The listing builds one solid part. Answer for the finished solid, in the listing's coordinates (mm). A direction names the side the tool comes from. Coordinates: 2 decimals unless noted, no trailing zeros. Order: outer loops, then holes, each group sorted by start corner. A loop starts at its lowest first (then second) coordinate and runs counter-clockwise, first axis right, second up. Notation, with made-up numbers: (63, 34.5) -> (91, 34.5) arc R11 cw to (91, 42.5) -> close; hole circle Ø11 at (-28, 22.5). An arc over 180 degrees is marked (long way). Write each question's results on one line, items separated by ' | '. Start each with the question number.
(1) The part is cut by section D-D, the plane z = 0.75. Give the vertices of the cut face in (x, y).
(2) The part is cut by section A-A, the plane z = 5.75. Give the vertices of the cut face in (x, y), then the cut area to 3 significant figures.
(3) Determine the mould class of faces 4 (the face through (-0.145, -2.073, 12.387)), 5 (the face through (-0.145, -2.073, -12.313)), 6 (the face through (17.66, -3.13, -0.92)), 7 (the face through (8, -6.35, 7)) for opening direction Y: +Y half, -Y half, draft (parallel to the pull), parting line (faces both ways), or undercut.
(4) Given pin 1 (1.9 mm diameter, centred on x = 18, y = -4, fed in from +Z), flat-ended and moving along its own axis, determine where the tip first touches the part or whether it passes through.
(5) The part is cut by section B-B, the plane x = 0. Give the vertices of the cut face in (y, z).
(6) A tool of negligible diameter and unlimited length cuts with its end or side. For faces 1 (the face through (-14.98, -3.13, 0.42)), 2 (the face through (19, -3, 5.231)), 3 (the face through (19, -3, -4.929)), from which of +Z, -Z, +X, -X, +Y, -Y can it reach the whole face along a straight path? Write none if from no direction.
(7) Straight lines are drawn through the part: L1, parallel to X at y = -1, z = 0.25; L2, parallel to Y at x = 0, z = -13; L3, parallel to Z at x = 9, y = -1. For each, find the intervals that lie inside material, in ascending order.
(8) The part is cut by section C-C, the plane y = -5. Give the vertices of the cut face in (x, z).
```python
from build123d import *

# Parameters (mm, degrees)
F0_R     = 1.7526
F0_R_2   = 9.779
F1_DEPTH = 6.35
F2_R     = 1.11125
F3_DEPTH = 25.4
F4_R     = 2.54
F5_R     = 2.54


with BuildPart() as f1:
    # F0 (on Front) → F1 (new body)
    with BuildSketch(Plane.XZ):
        with BuildLine():
            ThreePointArc((14.1521138842, -4.9292868255), (14.7760579092, -2.4996617102), (14.986, 0))
            ThreePointArc((14.986, 0), (14.7484924114, 2.6574739115), (14.0434979861, 5.2307131745))
            Line((14.0434979861, 5.2307131745), (14.0434979861, -4.9292868255))
            Line((14.0434979861, -4.9292868255), (14.1521138842, -4.9292868255))
        make_face()
        with BuildLine():
            ThreePointArc((14.0434979861, 5.2307131745), (14.7484924114, 2.6574739115), (14.986, 0))
            ThreePointArc((14.986, 0), (14.7760579092, -2.4996617102), (14.1521138842, -4.9292868255))
            Line((14.1521138842, -4.9292868255), (23.0350979861, -4.9292868255))
            Line((23.0350979861, -4.9292868255), (23.0350979861, 5.2307131745))
            Line((23.0350979861, 5.2307131745), (14.0434979861, 5.2307131745))
        make_face()
        with Locations((19.0472979861, 0.1507131745)):
            Circle(F0_R, mode=Mode.SUBTRACT)
        with BuildLine():
            Line((14.0434979861, -4.9292868255), (14.0434979861, 5.2307131745))
            ThreePointArc((14.0434979861, 5.2307131745), (-14.9851437159, -0.1601992956), (14.1521138842, -4.9292868255))
            Line((14.1521138842, -4.9292868255), (14.0434979861, -4.9292868255))
        make_face()
        Circle(F0_R_2, mode=Mode.SUBTRACT)
    extrude(amount=F1_DEPTH)

    # F2 (on Top) → F3 (cut, symmetric)
    with BuildSketch(Plane.XY):
        with Locations((0, -3.175)):
            Circle(F2_R)
    extrude(amount=F3_DEPTH, both=True, mode=Mode.SUBTRACT)

    # F4
    f4_edges = [f1.edges().sort_by_distance(p)[0] for p in [
        (14.043498, -3.175, 5.230713),
    ]]
    fillet(f4_edges, radius=F4_R)

    # F5
    f5_edges = [f1.edges().sort_by_distance(p)[0] for p in [
        (14.152114, -3.175, -4.929287),
    ]]
    fillet(f5_edges, radius=F5_R)


solid = f1.part
```
Established:
1) outline: (-14.97, -6.35) -> (-9.75, -6.35) -> (-9.75, 0) -> (-14.97, 0) -> close; (9.75, -6.35) -> (17.4, -6.35) -> (17.4, 0) -> (9.75, 0) -> close; (20.69, -6.35) -> (23.04, -6.35) -> (23.04, 0) -> (20.69, 0) -> close
2) outline: (-13.84, -6.35) -> (-7.91, -6.35) -> (-7.91, 0) -> (-13.84, 0) -> close; (7.91, -6.35) -> (14.17, -6.35) -> (14.17, 0) -> (7.91, 0) -> close | area: 77.4 mm^2
3) face 4: undercut | face 5: undercut | face 6: draft | face 7: -Y half
4) pin 1: stops at z = 5.23
5) outline: (-6.35, -14.99) -> (-4.29, -14.99) -> (-4.29, -9.78) -> (-6.35, -9.78) -> close; (-6.35, 9.78) -> (-4.29, 9.78) -> (-4.29, 14.99) -> (-6.35, 14.99) -> close; (-2.06, -14.99) -> (0, -14.99) -> (0, -9.78) -> (-2.06, -9.78) -> close; (-2.06, 9.78) -> (0, 9.78) -> (0, 14.99) -> (-2.06, 14.99) -> close
6) face 1: +Y, -Y | face 2: +Z, +X, +Y, -Y | face 3: -Z, +X, +Y, -Y
7) L1: x = -14.98 to -9.78, 9.78 to 17.3, 20.8 to 23.04 | L2: y = -6.35 to -4.29, -2.06 to 0 | L3: z = -11.98 to -3.82, 3.82 to 11.98
8) outline: (13.43, 6.64) arc R14.99 ccw (long way) to (13.56, -6.39) arc R2.54 cw to (15.85, -4.93) -> (23.04, -4.93) -> (23.04, 5.23) -> (15.71, 5.23) arc R2.54 cw to start; hole circle Ø19.56 at (0, 0); hole circle Ø3.51 at (19.05, 0.15)
